Source: CAD feature listing. Evaluate the final solid. Frame: model axes, mm. Round coordinates to 2 decimals unless told otherwise and drop trailing zeros. Write each loop counter-clockwise with the first axis right and the second up, starting at its lowest first coordinate (ties: lowest second). Pieces come first, ordered by that corner, then holes. Notation, with made-up numbers: M 7,5.5 L 18,5.5 A10 ccw 18,15.5 Z; hole C 29.25,62 d1. An arc over 180 degrees is marked long. Use a Markdown table: item, result.
```python
from build123d import *

# Parameters (mm, degrees)
SKETCH_1_W                 = 135.47
SKETCH_1_H                 = 60
EXTRUDE_1_DEPTH            = 1.6
HOLE_WIZARD_M3_1_OUTLINE_R = 1.6
HOLE_WIZARD_M3_1_DEPTH     = 1.6
FILLET_1_R                 = 1


# Read off the part's stored shape, not the designer's step: M3 すきま穴1
with BuildPart() as part:
    # ｽｹｯﾁ1 → ﾎﾞｽ - 押し出し1 (new body)
    with BuildSketch(Plane(origin=(0, 0, 0), x_dir=(1, 0, 0), z_dir=(0, 1, 0))):
        Rectangle(SKETCH_1_W, SKETCH_1_H)
    extrude(amount=EXTRUDE_1_DEPTH)

    # M3 すきま穴1 outline → M3 すきま穴1 (cut)
    with BuildSketch(Plane(origin=(0, 0, 0), x_dir=(1, 0, 0), z_dir=(0, 1, 0))):
        with Locations((64.735, 27)):
            Circle(HOLE_WIZARD_M3_1_OUTLINE_R)
        with Locations((-64.735, -27)):
            Circle(HOLE_WIZARD_M3_1_OUTLINE_R)
        with Locations((64.735, -27)):
            Circle(HOLE_WIZARD_M3_1_OUTLINE_R)
        with Locations((-64.735, 27)):
            Circle(HOLE_WIZARD_M3_1_OUTLINE_R)
    extrude(amount=HOLE_WIZARD_M3_1_DEPTH, mode=Mode.SUBTRACT)

    # ﾌｨﾚｯﾄ1
    fillet_1_edges = [part.edges().sort_by_distance(p)[0] for p in [
        (67.735, 0.8, 30),
        (-67.735, 0.8, 30),
        (-67.735, 0.8, -30),
        (67.735, 0.8, -30),
    ]]
    fillet(fillet_1_edges, radius=FILLET_1_R)


solid = part.part
```
Q1. Section A-A on z = -27. Return loops of the section in (x, y) (3 decimals).
Results are:
| item | result |
|---|---|
| outline | M -67.735,0 L -66.335,0 L -66.335,1.6 L -67.735,1.6 Z; M -63.135,0 L 63.135,0 L 63.135,1.6 L -63.135,1.6 Z; M 66.335,0 L 67.735,0 L 67.735,1.6 L 66.335,1.6 Z |
Q2. Line query: L1, parallel to X at y = 0.5, z = 27 (3 decimals); L2, parallel to X at y = 1.5, z = -26 (3 decimals). Output: solid intervals per line, ascending.
Results are:
| item | result |
|---|---|
| L1 | -67.735 to -66.335, -63.135 to 63.135, 66.335 to 67.735 |
| L2 | -67.735 to -65.984, -63.486 to 63.486, 65.984 to 67.735 |
Q3. First-contact query: pin 1 Ø12 at (x, z) = (-14, -15) entering from -Y. Flat tip, straight axial feed; report the tip coordinate or a pass-through.
Results are:
| item | result |
|---|---|
| pin 1 | y = 0 |
Q4. Mould query, pull axis Z, two halves, no side actions, for faces 1 (the flat face through (-1, 1.6, 0)), 2 (the cylindrical face through (63.137, 0.789, 26.93)). Classes: +Z half, -Z half, draft (parallel to the pull), parting line (faces both ways), or undercut.
Results are:
| item | result |
|---|---|
| face 1 | draft |
| face 2 | undercut |
